from build123d import *

# Parameters (mm, degrees)
SKETCH1_R                      = 15.875
SKETCH1_R_2                    = 12.7
SKETCH1_W                      = 101.6
SKETCH1_H                      = 3.81
BOSS_EXTRUDE1_DEPTH            = 25.4
F_5_16_0_3125_DIAMETER_HOLE1_D = 7.9375


with BuildPart() as part:
    # Sketch1 → Boss-Extrude1 (new body)
    # profile 1 of 4: a face of its own
    with BuildSketch(Plane.XY):
        Circle(SKETCH1_R)
        Circle(SKETCH1_R_2, mode=Mode.SUBTRACT)
    # profile 2 of 4: a face of its own
    with BuildSketch(Plane.XY):
        with BuildLine():
            ThreePointArc((-15.875, 0), (-20.524679849, -11.225320151), (-31.75, -15.875))
            Line((-31.75, -15.875), (3.4e-08, -15.875))
            ThreePointArc((3.4e-08, -15.875), (-11.225320139, -11.225320163), (-15.875, 0))
        make_face()
    # profile 3 of 4: a face of its own
    with BuildSketch(Plane.XY):
        with BuildLine():
            ThreePointArc((15.875, 0), (11.225320163, -11.225320139), (3.4e-08, -15.875))
            Line((3.4e-08, -15.875), (31.75, -15.875))
            ThreePointArc((31.75, -15.875), (20.524679849, -11.225320151), (15.875, 0))
        make_face()
    # profile 4 of 4: a face of its own
    with BuildSketch(Plane.XY):
        with Locations((0, -17.78)):
            Rectangle(SKETCH1_W, SKETCH1_H)
    extrude(amount=BOSS_EXTRUDE1_DEPTH)

    # 5/16 (0.3125) Diameter Hole1 (through all)
    with Locations(Plane(origin=(-41.275, -15.875, 12.7), x_dir=(1, 0, 0), z_dir=(0, 1, 0))):
        with Locations((0, 0)):
            f_5_16_0_3125_diameter_hole1 = Hole(F_5_16_0_3125_DIAMETER_HOLE1_D / 2)

    # Mirror1: 5/16 (0.3125) Diameter Hole1 across plane
    add(f_5_16_0_3125_diameter_hole1.mirror(Plane(origin=(0, 0, 0), x_dir=(0, 0, 1), z_dir=(1, 0, 0))), mode=Mode.SUBTRACT)


solid = part.part
CAD build for the part. Positions are in the model's coordinates, mm. A direction names the side the tool comes from. Coordinates: 2 decimals unless noted, no trailing zeros. Write each loop counter-clockwise with the first axis right and the second up, starting at its lowest first coordinate (ties: lowest second). Pieces come first, ordered by that corner, then holes. Notation, with made-up numbers: (60, -31.5) - (106, -31.5) arc R25 ccw to (106, -7.5) - close; hole circle Ø2 at (0, 63.5). An arc over 180 degrees is marked (long way). Use a Markdown table: item, result. Add a question column.
Item 1: Band-saw the part on A-A, the plane z = 12.7. Give the cut face in (x, y) (3 decimals).
Item 2: Flat gauge pins, fed straight in: pin 1 (5 mm diameter, centred on x = -5, y = -11.5, fed in from -Z); pin 2 (5.5 mm diameter, centred on x = -40.5, z = 11.5, fed in from +Y) (3 decimals); pin 3 (6 mm diameter, centred on y = 9.5, z = 19, fed in from -X). Where does each tip first touch, or does it go through?
Item 3: Band-saw the part on C-C, the plane z = 21.5. Give the cut face in (x, y) (3 decimals), and give its area (3 significant figures).
Item 4: Mould opens along Y. For faces 3 (the face through (-2.75, -12.4, 12.52)), 4 (the face through (-37, -15.875, 13)), 5 (the face through (43.409, -17.807, 9.354)) say: pulls with the +Y half, pulls with the -Y half, needs draft (parallel to the pull), parting line crosses it, or undercut.
Item 5: Drill centre lines: L1, parallel to Y at x = 0, z = 16.25 (3 decimals); L2, parallel to X at y = -17.5, z = 16.25; L3, parallel to X at y = 9, z = 21. Where is each one in solid material? Low to high. Write a range as from..to.
Item 6: Band-saw the part on D-D, the plane y = -6. Give the cut face in (x, z), and give its area (3 significant figures).
Item 7: Band-saw the part on B-B, the plane x = 0. Give the cut face in (y, z) (3 decimals), and give its area (3 significant figures).
Item 8: 3-axis set-ups, long thin cutter, end or side, ignore diameter. For faces 1 (the face through (37, -15.875, 13)), 2 (the face through (0, -15, 0)): which of +Z, -Z, +X, -X, +Y, -Y reach the whole face in a straight line?
Numbers:
| question | item | result |
|---|---|---|
| 1 | outline | (-50.8, -19.685) - (-45.244, -19.685) - (-45.244, -15.875) - (-50.8, -15.875) - close; (-37.306, -19.685) - (37.306, -19.685) - (37.306, -15.875) - (31.75, -15.875) arc R15.875 cw to (15.875, 0) arc R15.875 ccw to (-15.875, 0) arc R15.875 cw to (-31.75, -15.875) - (-37.306, -15.875) - close; (45.244, -19.685) - (50.8, -19.685) - (50.8, -15.875) - (45.244, -15.875) - close; hole circle Ø25.4 at (0, 0) |
| 2 | pin 1 | z = 0 |
| 2 | pin 2 | y = -15.875 |
| 2 | pin 3 | x = -14.48 |
| 3 | outline | (-50.8, -19.685) - (50.8, -19.685) - (50.8, -15.875) - (31.75, -15.875) arc R15.875 cw to (15.875, 0) arc R15.875 ccw to (-15.875, 0) arc R15.875 cw to (-31.75, -15.875) - (-50.8, -15.875) - close; hole circle Ø25.4 at (0, 0) |
| 3 | area | 888 mm2 |
| 4 | face 3 | undercut |
| 4 | face 4 | pulls with the +Y half |
| 4 | face 5 | needs draft |
| 5 | L1 | -19.685..-12.7, 12.7..15.875 |
| 5 | L2 | -50.8..-43.05, -39.5..39.5, 43.05..50.8 |
| 5 | L3 | -13.08..-8.96, 8.96..13.08 |
| 6 | outline | (-17.05, 0) - (-11.19, 0) - (-11.19, 25.4) - (-17.05, 25.4) - close; (11.19, 0) - (17.05, 0) - (17.05, 25.4) - (11.19, 25.4) - close |
| 6 | area | 298 mm2 |
| 7 | outline | (-19.685, 0) - (-12.7, 0) - (-12.7, 25.4) - (-19.685, 25.4) - close; (12.7, 0) - (15.875, 0) - (15.875, 25.4) - (12.7, 25.4) - close |
| 7 | area | 258 mm2 |
| 8 | face 1 | +Z, -Z, +X, +Y |
| 8 | face 2 | -Z, +X, -X, +Y, -Y |
